```python
from build123d import *

# Parameters (mm, degrees)
PAD_DEPTH   = 6
FILLET_R    = 1.5
FILLET001_R = 1


with BuildPart() as part:
    # Sketch → Pad (new body)
    with BuildSketch(Plane.XY):
        Polygon((0, 0), (0, 10), (30, 10), (30, 8), (70, 8), (70, 10), (100, 10), (100, 0), (70, 0), (70, 2), (30, 2), (30, 0), align=None)
    extrude(amount=PAD_DEPTH)

    # Fillet
    fillet_edges = [part.edges().sort_by_distance(p)[0] for p in [
        (70, 8, 3),
        (70, 2, 3),
        (30, 2, 3),
        (30, 8, 3),
    ]]
    fillet(fillet_edges, radius=FILLET_R)

    # Fillet001
    fillet001_edges = [part.edges().sort_by_distance(p)[0] for p in [
        (30, 10, 3),
        (30, 0, 3),
        (70, 0, 3),
        (70, 10, 3),
    ]]
    fillet(fillet001_edges, radius=FILLET001_R)


solid = part.part
```
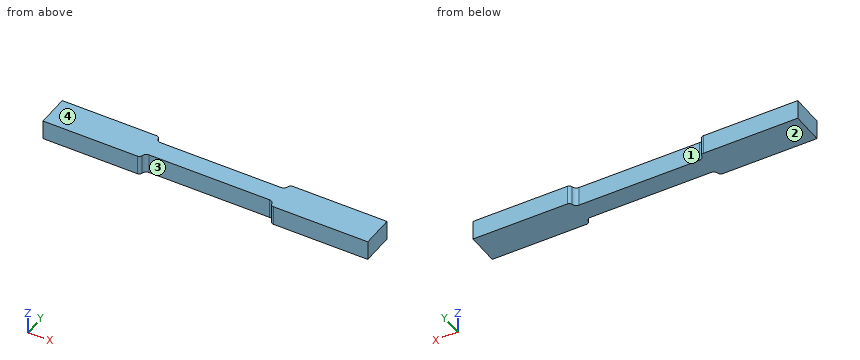
CAD build for the part. Positions are in the model's coordinates, mm. Face numbers are marked on the shaded views. A direction names the side the tool comes from. Coordinates: 2 decimals unless noted, no trailing zeros. Order: outer loops, then holes, each group sorted by start corner. A loop starts at its lowest first (then second) coordinate and runs counter-clockwise, first axis right, second up.
(1) Drill centre lines: L1, parallel to X at y = 1.5, z = 3; L2, parallel to X at y = 0.75, z = 1; L3, parallel to Y at x = 49.5, z = 2.5. Where is each one in solid material? Low to high.
Solution:
L1: x = 0 to 30.38, 69.62 to 100
L2: x = 0 to 30.02, 69.98 to 100
L3: y = 2 to 8
(2) Pin check, flat tips, straight feed: pin 1 Ø1.5 at (y, z) = (6.5, 5) entering from -X; pin 2 Ø1.8 at (x, z) = (58.5, 3.5) entering from +Y. Stop position of each tip, or through.
Solution:
pin 1: stops at x = 0
pin 2: stops at y = 8
(3) Saw through at A-A, the plane x = 48.5. Write the cut outline in (y, z), and give its area (3 significant figures).
Solution:
outline: (2, 0) - (8, 0) - (8, 6) - (2, 6) - close
area: 36.0 mm2
(4) Mould opens along X. For the marked faces 3 and 4 say: released by +X, released by -X, zero draft, split by the parting line, or undercut.
Solution:
face 3: undercut
face 4: zero draft
(5) Which spindle directions (+Z, -Z, +X, -X, +Y, -Y) get a long thin tool onto all of the face, cutting with end or side? Do the marked faces 1 and 2. Say none if no direction does.
Solution:
face 1: +Z, -Z, +Y
face 2: -Z, +X, -X, +Y, -Y
